```python
from build123d import *

# Parameters (mm, degrees)
GASKET_START = -1.5
GASKET_DEPTH = 1.5


with BuildPart() as part:
    # Sketch1 → Gasket (new body)
    with BuildSketch(Plane(origin=(0, 0, 0), x_dir=(1, 0, 0), z_dir=(0, 1, 0)).offset(GASKET_START)):
        with BuildLine():
            Line((-41, -23.9), (41, -23.9))
            ThreePointArc((41, -23.9), (45.87903679, -21.87903679), (47.9, -17))
            Line((47.9, -17), (47.9, 17))
            ThreePointArc((47.9, 17), (45.87903679, 21.87903679), (41, 23.9))
            Line((41, 23.9), (-41, 23.9))
            ThreePointArc((-41, 23.9), (-45.87903679, 21.87903679), (-47.9, 17))
            Line((-47.9, 17), (-47.9, -17))
            ThreePointArc((-47.9, -17), (-45.87903679, -21.87903679), (-41, -23.9))
        make_face()
        with BuildLine():
            Line((-41, -22.1), (41, -22.1))
            ThreePointArc((41, -22.1), (44.606244584, -20.606244584), (46.1, -17))
            Line((46.1, -17), (46.1, 17))
            ThreePointArc((46.1, 17), (44.606244584, 20.606244584), (41, 22.1))
            Line((41, 22.1), (-41, 22.1))
            ThreePointArc((-41, 22.1), (-44.606244584, 20.606244584), (-46.1, 17))
            Line((-46.1, 17), (-46.1, -17))
            ThreePointArc((-46.1, -17), (-44.606244584, -20.606244584), (-41, -22.1))
        make_face(mode=Mode.SUBTRACT)
    extrude(amount=GASKET_DEPTH)


solid = part.part
```
Geometry check sheet. Reference: the model listing, model coordinates, mm. A direction names the side the tool comes from. Round coordinates to 2 decimals unless told otherwise and drop trailing zeros. Write each loop counter-clockwise with the first axis right and the second up, starting at its lowest first coordinate (ties: lowest second). Pieces come first, ordered by that corner, then holes. Notation, with made-up numbers: (-18, 44) - (31, 44) arc R26 cw to (31, 83) - close; hole circle Ø8 at (48, 4.25). An arc over 180 degrees is marked (long way). Write each question's results on one line, items separated by ' | '.
(1) Sectioned sample at A-A, the plane z = 0.5. Enter the section's corners in (x, y).
Computed:
outline: (-47.9, -1.5) - (-46.1, -1.5) - (-46.1, 0) - (-47.9, 0) - close; (46.1, -1.5) - (47.9, -1.5) - (47.9, 0) - (46.1, 0) - close
(2) Sectioned sample at B-B, the plane y = -0.75. Enter the section's corners in (x, z), plus the area to 3 significant figures.
Computed:
outline: (-47.9, -17) arc R6.9 ccw to (-41, -23.9) - (41, -23.9) arc R6.9 ccw to (47.9, -17) - (47.9, 17) arc R6.9 ccw to (41, 23.9) - (-41, 23.9) arc R6.9 ccw to (-47.9, 17) - close; hole (-46.1, -17) arc R5.1 ccw to (-41, -22.1) - (41, -22.1) arc R5.1 ccw to (46.1, -17) - (46.1, 17) arc R5.1 ccw to (41, 22.1) - (-41, 22.1) arc R5.1 ccw to (-46.1, 17) - close | area: 485 mm^2
(3) Set-up check for faces 1 (the face through (-44.646, -0.76, 20.566)), 2 (the face through (45.83, -0.76, 21.93)): record each of +Z, -Z, +X, -X, +Y, -Y from which the full face is reachable in a straight line by a thin tool's end or side.
Computed:
face 1: +Y, -Y | face 2: +Z, +X, +Y, -Y
(4) Sectioned sample at C-C, the plane x = 20. Enter the section's corners in (y, z).
Computed:
outline: (-1.5, -23.9) - (0, -23.9) - (0, -22.1) - (-1.5, -22.1) - close; (-1.5, 22.1) - (0, 22.1) - (0, 23.9) - (-1.5, 23.9) - close
(5) Draft check along X on faces 3 (the face through (44.566, -0.76, 20.646)), 4 (the face through (-11, 0, 23)), 5 (the face through (-44.566, -0.76, -20.646)), 6 (the face through (-45.93, -0.76, 21.83)). Enter one of: pulls with the +X half, pulls with the -X half, needs draft (parallel to the pull), parting line crosses it, or undercut.
Computed:
face 3: undercut | face 4: needs draft | face 5: undercut | face 6: pulls with the -X half
(6) Thickness scan on probe 1 along Z at (x, y) = (38, -0.35); probe 2 along X at (y, z) = (-0.8, -8.5); probe 3 along X at (y, z) = (-0.45, -18.5). Record the ranges inside material, lowest first. Write a range as from..to.
Computed:
probe 1: z = -23.9..-22.1, 22.1..23.9 | probe 2: x = -47.9..-46.1, 46.1..47.9 | probe 3: x = -47.73..-45.87, 45.87..47.73
